```python
from build123d import *

# Parameters (mm, degrees)
BOSS_EXTRUDE1_DEPTH          = 50.8
F_39_0_0995_DIAMETER_HOLE1_D = 2.5273
F_46_0_081_DIAMETER_HOLE1_D  = 2.0574
SKETCH9_R                    = 5.489854512
CUT_EXTRUDE1_DEPTH           = 73.955945611


with BuildPart() as part:
    # Sketch4 → Boss-Extrude1 (new body)
    with BuildSketch(Plane.XY):
        Polygon((0, 0), (0, 50.8), (3.302, 50.8), (3.302, 3.302), (12.7, 3.302), (12.7, 0), align=None)
    extrude(amount=BOSS_EXTRUDE1_DEPTH)

    # #39 (0.0995) Diameter Hole1 (through all)
    with Locations(Plane(origin=(0, 0, 0), x_dir=(-1, 0, 0), z_dir=(0, -1, 0))):
        with Locations((-9.908705213, -43.283410028), (-9.908705213, -26.281703485), (-9.908705213, -9.270127085)):
            Hole(F_39_0_0995_DIAMETER_HOLE1_D / 2)

    # #46 (0.081) Diameter Hole1 (through all)
    with Locations(Plane.ZY):
        with Locations((38.924052109, 20.132703071), (33.256732001, 22.45014951), (30.924052109, 28.132703071), (33.256732001, 33.754608506), (38.924052109, 36.096767323), (44.576588318, 33.763667384), (46.921652769, 28.101604064), (44.576588318, 22.45014951)):
            Hole(F_46_0_081_DIAMETER_HOLE1_D / 2)

    # Sketch9 → Cut-Extrude1 (cut, through all)
    with BuildSketch(Plane.ZY):
        with Locations((38.924052109, 28.132703071)):
            Circle(SKETCH9_R)
        Polygon((0, 19.05), (31.75, 50.8), (0, 50.8), align=None)
    extrude(amount=-CUT_EXTRUDE1_DEPTH, mode=Mode.SUBTRACT)


solid = part.part
```
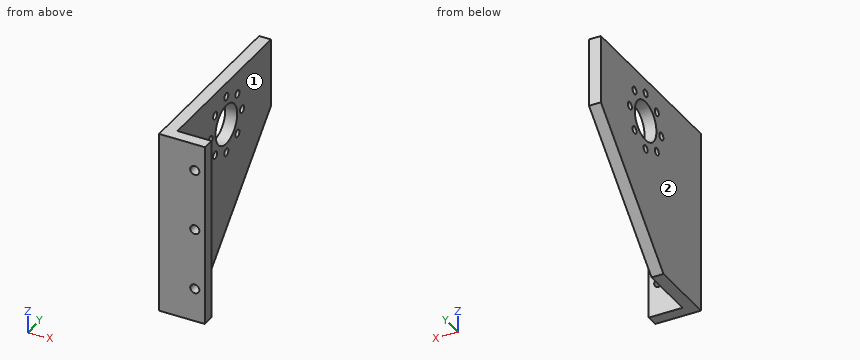
Source: CAD feature listing. Evaluate the final solid. Frame: model axes, mm. Face numbers are marked on the shaded views. A direction names the side the tool comes from. Coordinates: 2 decimals unless noted, no trailing zeros. Loops run counter-clockwise (first coordinate to the right, second up) from the corner with the lowest first, then second, coordinate; pieces in that order, holes last. Notation, with made-up numbers: M -18,80 L 19,80 A8 cw 19,88 Z; hole C 53,75 d4. An arc over 180 degrees is marked long. Use CSV: the item, a comma, the result in double quotes.
(1) Cut plane B-B on x = 10. Return loops of the section in (y, z), and give its area (3 significant figures).
Answers follow:
outline,"M 0,0 L 3.3,0 L 3.3,8.01 L 0,8.01 Z; M 0,10.53 L 3.3,10.53 L 3.3,25.02 L 0,25.02 Z; M 0,27.54 L 3.3,27.54 L 3.3,42.02 L 0,42.02 Z; M 0,44.54 L 3.3,44.54 L 3.3,50.8 L 0,50.8 Z"
area,"143 mm²"
(2) Cut plane C-C on z = 31. Return loops of the section in (x, y), and give its area (3 significant figures).
Answers follow:
outline,"M 0,0 L 12.7,0 L 12.7,3.3 L 3.3,3.3 L 3.3,27.11 L 0,27.11 Z; M 0,29.16 L 3.3,29.16 L 3.3,50.05 L 0,50.05 Z"
area,"190 mm²"
(3) Reachability of the marked faces 1 and 2 from +Z, -Z, +X, -X, +Y, -Y: full face, straight path, thin tool, end or side. Return the list, or none.
Answers follow:
face 1,"+Z, -Z, +X, +Y"
face 2,"+Z, -Z, -X, +Y, -Y"
(4) Contact query for flat-ended pins moving along their axis: pin 1 (4 mm diameter, centred on x = 7.5, z = 20, fed in from -Y); pin 2 (2 mm diameter, centred on x = 9.91, z = 9.27, fed in from -Y); pin 3 (7.5 mm diameter, centred on x = 7.5, z = 14.5, fed in from +Y); pin 4 (17.5 mm diameter, centred on y = 28.13, z = 38.92, fed in from +X). Output: stop coordinate, or through.
Answers follow:
pin 1,"y = 0"
pin 2,"through"
pin 3,"y = 3.3"
pin 4,"x = 3.3"
(5) Cut plane D-D on z = 17.5. Return loops of the section in (x, y).
Answers follow:
outline,"M 0,0 L 12.7,0 L 12.7,3.3 L 3.3,3.3 L 3.3,36.55 L 0,36.55 Z"
(6) Line query: line 1 (Y direction, x = 0.75, z = 45.5); line 2 (Y direction, x = 11.5, z = 14). Output: solid intervals per line, ascending. Write a range as [from, to].
Answers follow:
line 1,"[0, 22], [22.9, 33.31], [34.22, 50.8]"
line 2,"[0, 3.3]"
(7) Cut plane A-A on y = 25. Return loops of the section in (x, z), and give its area (3 significant figures).
Answers follow:
outline,"M 0,5.95 L 3.3,5.95 L 3.3,34.42 L 0,34.42 Z; M 0,43.43 L 3.3,43.43 L 3.3,50.8 L 0,50.8 Z"
area,"118 mm²"
